The model under review builds one solid part; all positions refer to its coordinate system, in mm. A direction names the side the tool comes from. Coordinates: 2 decimals unless noted, no trailing zeros. Write each loop counter-clockwise with the first axis right and the second up, starting at its lowest first coordinate (ties: lowest second). Pieces come first, ordered by that corner, then holes.
```python
from build123d import *

# Parameters (mm, degrees)
SKETCH3_W           = 149
SKETCH3_H           = 141.12
BOSS_EXTRUDE1_DEPTH = 4
SKETCH5_W           = 67
SKETCH5_H           = 30.2
SKETCH5_H_2         = 36.35
BOSS_EXTRUDE2_DEPTH = 14.5
FILLET1_R           = 2
SKETCH6_W           = 149
SKETCH6_H           = 12
BOSS_EXTRUDE3_DEPTH = 10.5
FILLET2_R           = 2


with BuildPart() as part:
    # Sketch3 → Boss-Extrude1 (new body)
    with BuildSketch(Plane(origin=(0, 0, 0), x_dir=(1, 0, 0), z_dir=(0, 1, 0))):
        with Locations((74.5, -70.56)):
            Rectangle(SKETCH3_W, SKETCH3_H)
    extrude(amount=BOSS_EXTRUDE1_DEPTH)

    # Sketch5 → Boss-Extrude2 (add)
    # profile 1 of 6: a face of its own
    with BuildSketch(Plane(origin=(0, 4, 0), x_dir=(1, 0, 0), z_dir=(0, 1, 0))):
        with Locations((33.5, -23.8)):
            Rectangle(SKETCH5_W, SKETCH5_H)
        with BuildLine():
            ThreePointArc((13, -27.9), (9.9, -24.8), (13, -21.7))
            Line((13, -21.7), (41, -21.7))
            ThreePointArc((41, -21.7), (44.1, -24.8), (41, -27.9))
            Line((41, -27.9), (13, -27.9))
        make_face(mode=Mode.SUBTRACT)
    # profile 2 of 6: a face of its own
    with BuildSketch(Plane(origin=(0, 4, 0), x_dir=(1, 0, 0), z_dir=(0, 1, 0))):
        with Locations((115.5, -18.175)):
            Rectangle(SKETCH5_W, SKETCH5_H_2)
        with BuildLine():
            ThreePointArc((97, -25.35), (93.9, -22.25), (97, -19.15))
            Line((97, -19.15), (125, -19.15))
            ThreePointArc((125, -19.15), (128.1, -22.25), (125, -25.35))
            Line((125, -25.35), (97, -25.35))
        make_face(mode=Mode.SUBTRACT)
    # profile 3 of 6: a face of its own
    with BuildSketch(Plane(origin=(0, 4, 0), x_dir=(1, 0, 0), z_dir=(0, 1, 0))):
        with Locations((33.5, -63.9)):
            Rectangle(SKETCH5_W, SKETCH5_H)
        with BuildLine():
            ThreePointArc((13, -68), (9.9, -64.9), (13, -61.8))
            Line((13, -61.8), (41, -61.8))
            ThreePointArc((41, -61.8), (44.1, -64.9), (41, -68))
            Line((41, -68), (13, -68))
        make_face(mode=Mode.SUBTRACT)
    # profile 4 of 6: a face of its own
    with BuildSketch(Plane(origin=(0, 4, 0), x_dir=(1, 0, 0), z_dir=(0, 1, 0))):
        with Locations((115.5, -61.35)):
            Rectangle(SKETCH5_W, SKETCH5_H)
        with BuildLine():
            ThreePointArc((97, -65.45), (93.9, -62.35), (97, -59.25))
            Line((97, -59.25), (125, -59.25))
            ThreePointArc((125, -59.25), (128.1, -62.35), (125, -65.45))
            Line((125, -65.45), (97, -65.45))
        make_face(mode=Mode.SUBTRACT)
    # profile 5 of 6: a face of its own
    with BuildSketch(Plane(origin=(0, 4, 0), x_dir=(1, 0, 0), z_dir=(0, 1, 0))):
        with Locations((33.5, -104)):
            Rectangle(SKETCH5_W, SKETCH5_H)
        with BuildLine():
            ThreePointArc((13, -108.1), (9.9, -105), (13, -101.9))
            Line((13, -101.9), (41, -101.9))
            ThreePointArc((41, -101.9), (44.1, -105), (41, -108.1))
            Line((41, -108.1), (13, -108.1))
        make_face(mode=Mode.SUBTRACT)
    # profile 6 of 6: a face of its own
    with BuildSketch(Plane(origin=(0, 4, 0), x_dir=(1, 0, 0), z_dir=(0, 1, 0))):
        with Locations((115.5, -101.45)):
            Rectangle(SKETCH5_W, SKETCH5_H)
        with BuildLine():
            ThreePointArc((97, -105.55), (93.9, -102.45), (97, -99.35))
            Line((97, -99.35), (125, -99.35))
            ThreePointArc((125, -99.35), (128.1, -102.45), (125, -105.55))
            Line((125, -105.55), (97, -105.55))
        make_face(mode=Mode.SUBTRACT)
    extrude(amount=-BOSS_EXTRUDE2_DEPTH)

    # Fillet1
    fillet1_edges = [part.edges().sort_by_distance(p)[0] for p in [
        (67, -5.25, 48.8),
        (67, -5.25, 79),
        (0, -5.25, 79),
        (0, -5.25, 48.8),
        (82, -5.25, 46.25),
        (149, -5.25, 46.25),
        (149, -5.25, 76.45),
        (82, -5.25, 76.45),
        (67, -5.25, 88.9),
        (67, -5.25, 119.1),
        (0, -5.25, 119.1),
        (0, -5.25, 88.9),
        (82, -5.25, 86.35),
        (149, -5.25, 86.35),
        (149, -5.25, 116.55),
        (82, -5.25, 116.55),
        (67, -5.25, 8.7),
        (67, -5.25, 38.9),
        (0, -5.25, 38.9),
        (0, -5.25, 8.7),
        (82, -5.25, 0),
        (149, -5.25, 36.35),
        (82, -5.25, 36.35),
        (149, -3.25, 0),
    ]]
    fillet(fillet1_edges, radius=FILLET1_R)

    # Sketch6 → Boss-Extrude3 (add)
    with BuildSketch(Plane.XZ):
        with Locations((74.5, 135.12)):
            Rectangle(SKETCH6_W, SKETCH6_H)
    extrude(amount=BOSS_EXTRUDE3_DEPTH)

    # Fillet2
    fillet2_edges = [part.edges().sort_by_distance(p)[0] for p in [
        (0, -5.25, 129.12),
        (149, -5.25, 129.12),
        (0, 2, 0),
        (149, -3.25, 141.12),
        (0, -3.25, 141.12),
    ]]
    fillet(fillet2_edges, radius=FILLET2_R)


solid = part.part
```
Item 1: Take a section at D-D, the plane x = 102. Write out the cut boundary in (y, z), plus the area to 3 significant figures.
Solved:
outline: (-10.5, 0) - (4, 0) - (4, 141.12) - (-10.5, 141.12) - (-10.5, 129.12) - (0, 129.12) - (0, 116.55) - (-10.5, 116.55) - (-10.5, 105.55) - (0, 105.55) - (0, 99.35) - (-10.5, 99.35) - (-10.5, 86.35) - (0, 86.35) - (0, 76.45) - (-10.5, 76.45) - (-10.5, 65.45) - (0, 65.45) - (0, 59.25) - (-10.5, 59.25) - (-10.5, 46.25) - (0, 46.25) - (0, 36.35) - (-10.5, 36.35) - (-10.5, 25.35) - (0, 25.35) - (0, 19.15) - (-10.5, 19.15) - close
area: 1,510 mm2
Item 2: Take a section at B-B, the plane y = -7. Count the separate pieces of the cut face and the enclosed holes in it, plus the area to 3 significant figures.
Solved:
separate pieces: 7
enclosed holes: 6
area: 13,100 mm2
Item 3: Mouldability with a two-part tool opening along Z and no side actions: class faces 6 (the face through (33, -5, 8.7)), 7 (the face through (115, -5, 36.35)), 8 (the face through (73, 4, 70)), 9 (the face through (115, -5, 76.45)) as pulls with the +Z half, pulls with the -Z half, needs draft (parallel to the pull), parting line crosses it, or undercut.
Solved:
face 6: pulls with the -Z half
face 7: undercut
face 8: needs draft
face 9: undercut
Item 4: Machinability: for faces 1 (the face through (82, -5, 62)), 2 (the face through (93.9, -5.2, 22.3)), 3 (the face through (33, -10.5, 100)), 4 (the face through (115, -5, 86.35)), 5 (the face through (33, -5, 48.8)), which of the approach directions +Z, -Z, +X, -X, +Y, -Y give a long, thin tool a straight path to every point of the face, cutting with its end or side? Answer none if there is none.
Solved:
face 1: -Z, -Y
face 2: -Y
face 3: +Z, -Z, +X, -X, -Y
face 4: +X, -X, -Y
face 5: -X, -Y
Item 5: To check wall thickness, follow line 1 along Z through (x, y) = (63, -0.25); line 2 along Z through (x, y) = (130.5, -9.25); line 3 along X through (y, z) = (-7.5, 96.5). State the ranges of each line that lie inside material, in increasing order.
Solved:
line 1: z = 8.7 to 38.9, 48.8 to 79, 88.9 to 119.1, 129.12 to 141.12
line 2: z = 0 to 36.35, 46.25 to 76.45, 86.35 to 116.55, 129.12 to 141.12
line 3: x = 0 to 67, 82 to 149
Item 6: For pin 1 (5 mm diameter, centred on x = 30, y = -7, fed in from -Z); pin 2 (3 mm diameter, centred on x = 28.5, z = 63.5, fed in from -Y), all flat-tipped, find the tip position at first contact; note any pin that passes through.
Solved:
pin 1: stops at z = 8.7
pin 2: stops at y = 0
Item 7: Take a section at C-C, the plane z = 110. Write out the cut boundary in (x, y), plus the area to 3 significant figures.
Solved:
outline: (0, -10.5) - (67, -10.5) - (67, 0) - (82, 0) - (82, -10.5) - (149, -10.5) - (149, 4) - (0, 4) - close
area: 2,000 mm2
